Source: three-view drawing plus pictorial views. Frame: mm from the lowest corner of the part. Give positions to 0.01 mm unless a question says otherwise; leave off trailing zeros. Order: outer loops, then holes, each group sorted by start corner. A loop starts at its lowest first (then second) coordinate and runs counter-clockwise, first axis right, second up. Notation, with made-up numbers: M 59,34.25 L 111,34.25 A15 ccw 111,43.25 Z; hole C 60.5,9 d6. An arc over 180 degrees is marked long. One line per item, written item: value. Start each with the question number.
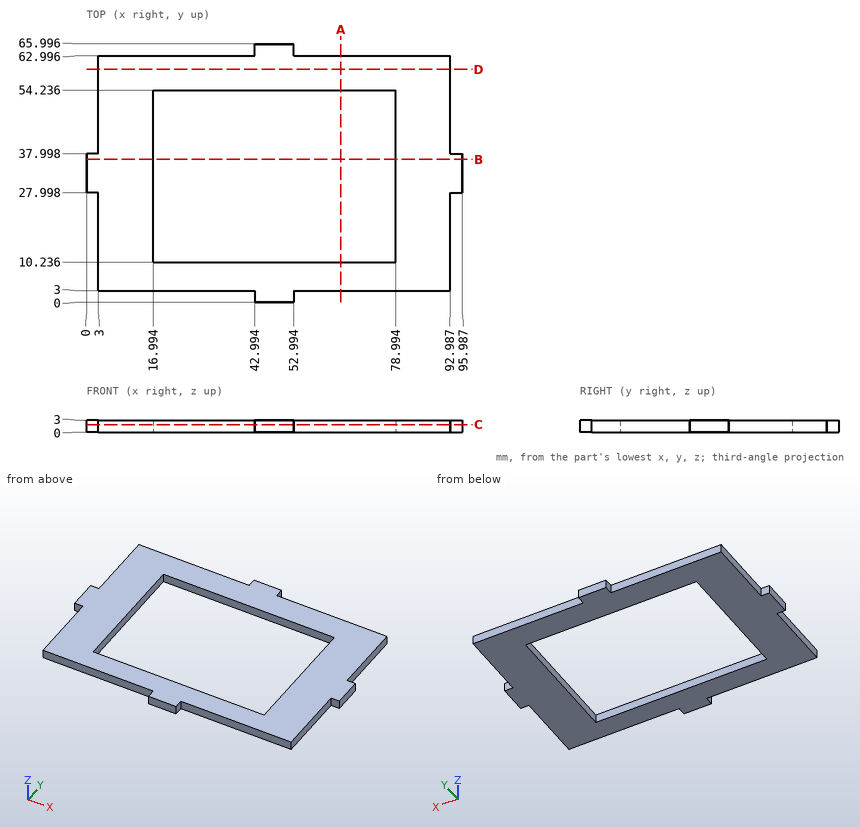
Q1. Section query D-D on y = 59.5. Return loops of the section in (x, z), and give its area (3 significant figures).
Q2. Section query B-B on y = 36.5. Return loops of the section in (x, z).
Q3. Section query A-A on x = 65. Return loops of the section in (y, z) (1 decimal).
Q4. Section query C-C on z = 1.9. Return loops of the section in (x, y) (1 decimal).
Q5. Contact query for flat-ended pins moving along their axis: pin 1 (5 mm diameter, centred on x = 77, y = 49, fed in from +Z); pin 2 (0.9 mm diameter, centred on x = 64, z = 1.5, fed in from +Y); pin 3 (0.9 mm diameter, centred on x = 1, z = 1.5, fed in from +Y). Output: stop coordinate, or through.
Q6. Ray query, line 1 along X through (y, z) = (38.5, 0.85); line 2 along Y through (x, z) = (57, 1.25) (1 decimal); line 3 along X through (y, z) = (33.5, 2.85). Return the intervals inside material, ascending. Write a range as [from, to].
Results below:
1. outline: M 3,0 L 92.99,0 L 92.99,3 L 3,3 Z
1. area: 270 mm2
2. outline: M 0,0 L 16.99,0 L 16.99,3 L 0,3 Z; M 78.99,0 L 95.99,0 L 95.99,3 L 78.99,3 Z
3. outline: M 3,0 L 10.2,0 L 10.2,3 L 3,3 Z; M 54.2,0 L 63,0 L 63,3 L 54.2,3 Z
4. outline: M 0,28 L 3,28 L 3,3 L 43,3 L 43,0 L 53,0 L 53,3 L 93,3 L 93,28 L 96,28 L 96,38 L 93,38 L 93,63 L 53,63 L 53,66 L 43,66 L 43,63 L 3,63 L 3,38 L 0,38 Z; hole M 17,10.2 L 79,10.2 L 79,54.2 L 17,54.2 Z
5. pin 1: z = 3
5. pin 2: y = 63
5. pin 3: y = 38
6. line 1: [3, 16.99], [78.99, 92.99]
6. line 2: [3, 10.2], [54.2, 63]
6. line 3: [0, 16.99], [78.99, 95.99]
